from build123d import *

# Parameters (mm, degrees)
F0_R      = 11.5
F1_DEPTH  = 2
F3_DEPTH  = 5
F5_DEPTH  = 10.5
F6_W      = 0.8
F6_H      = 5
F7_DEPTH  = 5
F8_R      = 8.8
F9_DEPTH  = 6
F11_R     = 2
F12_SIZE  = 0.75
F13_R     = 0.9
F14_DEPTH = 21.9495823706


# Not quite as in the source:
# - a fillet or chamfer that OpenCascade refuses, or shapes differently, is made with other operations: its cross-section is extruded or revolved along the edge and cut away or added


with BuildPart() as f1:
    # F0 (on Top) → F1 (new body)
    with BuildSketch(Plane.XY):
        Circle(F0_R)
    extrude(amount=F1_DEPTH)

    # F2 (on face) → F3 (join)
    with BuildSketch(Plane(origin=(0, 0, 0), x_dir=(1, 0, 0), z_dir=(0, 0, -1))):
        with BuildLine():
            Line((-9.05, -2), (-9.05, -3.6276714294))
            ThreePointArc((-9.05, -3.6276714294), (0, -9.75), (9.05, -3.6276714294))
            Line((9.05, -3.6276714294), (9.05, -2))
            Line((9.05, -2), (9.05, 2))
            Line((9.05, 2), (9.05, 3.6276714294))
            ThreePointArc((9.05, 3.6276714294), (5.8706571109, 7.7844643416), (1, 9.6985823706))
            Line((1, 9.6985823706), (1, 10.4485823706))
            Line((1, 10.4485823706), (-1, 10.4485823706))
            Line((-1, 10.4485823706), (-1, 9.6985823706))
            ThreePointArc((-1, 9.6985823706), (-5.8706571109, 7.7844643416), (-9.05, 3.6276714294))
            Line((-9.05, 3.6276714294), (-9.05, 2))
            Line((-9.05, 2), (-9.05, -2))
        make_face()
        with BuildLine():
            Line((-9.542667342, -2), (-9.05, -2))
            Line((-9.05, -2), (-9.05, 2))
            Line((-9.05, 2), (-9.542667342, 2))
            ThreePointArc((-9.542667342, 2), (-9.75, 0), (-9.542667342, -2))
        make_face()
        with BuildLine():
            Line((9.05, 2), (9.05, -2))
            Line((9.05, -2), (9.542667342, -2))
            ThreePointArc((9.542667342, -2), (9.75, 0), (9.542667342, 2))
            Line((9.542667342, 2), (9.05, 2))
        make_face()
    extrude(amount=F3_DEPTH)

    # F4 (on face) → F5 (join)
    with BuildSketch(Plane(origin=(0, 0, -5), x_dir=(1, 0, 0), z_dir=(0, 0, -1))):
        with BuildLine():
            Line((6.5, 5.35), (-6.5, 5.35))
            ThreePointArc((-6.5, 5.35), (-7.9142135624, 4.7642135624), (-8.5, 3.35))
            Line((-8.5, 3.35), (-8.5, -3.35))
            ThreePointArc((-8.5, -3.35), (-7.9142135624, -4.7642135624), (-6.5, -5.35))
            Line((-6.5, -5.35), (6.5, -5.35))
            ThreePointArc((6.5, -5.35), (7.9142135624, -4.7642135624), (8.5, -3.35))
            Line((8.5, -3.35), (8.5, 3.35))
            ThreePointArc((8.5, 3.35), (7.9142135624, 4.7642135624), (6.5, 5.35))
        make_face()
    extrude(amount=F5_DEPTH)

    # F6 (on face) → F7 (cut)
    with BuildSketch(Plane(origin=(0, 0, -15.5), x_dir=(1, 0, 0), z_dir=(0, 0, -1))):
        Rectangle(F6_W, F6_H)
        with Locations((-7.1, 0)):
            Rectangle(F6_W, F6_H)
        with Locations((7.1, 0)):
            Rectangle(F6_W, F6_H)
    extrude(amount=-F7_DEPTH, mode=Mode.SUBTRACT)

    # F8 (on face) → F9 (cut)
    with BuildSketch(Plane.XY.offset(2)):
        Circle(F8_R)
    extrude(amount=-F9_DEPTH, mode=Mode.SUBTRACT)

    # F10: chamfer of 2.8 x 1 on 1 edges, made by hand

    # F10_s1 → F10_t2 (revolve, cut)
    with BuildSketch(Plane.XZ):
        Polygon((11.5, 1), (8.7, 2), (11.5, 2), align=None)
    revolve(axis=Axis((0, 0, 2), (0, 0, 1)), mode=Mode.SUBTRACT)

    # F11
    f11_edges = [f1.edges().sort_by_distance(p)[0] for p in [
        (-9.05, 3.627671, -2.5),
        (-9.05, -3.627671, -2.5),
        (9.05, -3.627671, -2.5),
        (9.05, 3.627671, -2.5),
    ]]
    fillet(f11_edges, radius=F11_R)

    # F12
    f12_edges = [f1.edges().sort_by_distance(p)[0] for p in [
        (0, -10.448582, -5),
    ]]
    chamfer(f12_edges, length=F12_SIZE)

    # F13 (on face) → F14 (cut, through all)
    with BuildSketch(Plane.XZ.offset(10.4485823706)):
        with Locations((0, -1.4)):
            Circle(F13_R)
    extrude(amount=-F14_DEPTH, mode=Mode.SUBTRACT)


solid = f1.part
The listing builds one solid part. Answer for the finished solid, in the listing's coordinates (mm). A direction names the side the tool comes from. Coordinates: 2 decimals unless noted, no trailing zeros. Loops run counter-clockwise (first coordinate to the right, second up) from the corner with the lowest first, then second, coordinate; pieces in that order, holes last. Notation, with made-up numbers: (-39, 82.25) -> (6, 82.25) arc R19 cw to (6, 91.25) -> close; hole circle Ø11 at (29.25, -29.5). An arc over 180 degrees is marked (long way). Write item = value, one per line. Start each with the question number.
1) A cutting plane is placed at B-B (z = -1.4). Give the vertices of the cut face in (x, y), then the cut area to 3 significant figures.
2) A cutting plane is placed at A-A (x = 0). Count the separate pieces of the cut face and the enclosed holes in it, then the cut area to 3 significant figures.
3) The mould has two halves that part along X. Classify faces 1 (the face through (-0.16, 9.75, -2.46)), 2 (the face through (9.003, -3.65, -2.535)), 3 (the face through (0, 5.35, -10)), 4 (the face through (-6.7, 0, -13)): released by +X, released by -X, zero draft, split by the parting line, or undercut.
4) Straight lines are drawn through the part: line 1 (Z direction, x = 5, y = -3); line 2 (X direction, y = -0.5, z = -6.5); line 3 (Y direction, x = 2.5, z = -13). For each, find the intervals that lie inside material, in ascending order. Write a range as from..to.
5) Given pin 1 Ø0.9 at (x, z) = (-7.5, -13.5) entering from +Y; pin 2 Ø5 at (y, z) = (-5.5, -6.5) entering from -X; pin 3 Ø1.5 at (y, z) = (-0.5, -11.5) entering from +X, each flat-ended and moving along its own axis, determine where each tip first touches the part or whether it passes through.
6) A tool of negligible diameter and unlimited length cuts with its end or side. For faces 5 (the face through (5.74, -7.88, -2.46)), 6 (the face through (-1.146, 8.725, -0.976)), 7 (the face through (7, 2.5, -13)), from which of +Z, -Z, +X, -X, +Y, -Y can it reach the whole face along a straight path? Write none if from no direction.
7) A cutting plane is placed at C-C (y = 0). Give the vertices of the cut face in (x, z).
Responses:
q1.outline = (-9.54, -2) -> (-9.05, -2) -> (-9.05, -3.22) arc R2 ccw to (-8.87, -4.05) arc R9.75 ccw to (-1, -9.7) -> (-1, -10.45) -> (-0.9, -10.45) -> (-0.9, -8.75) arc R8.8 cw to (-0.9, 8.75) -> (-0.9, 9.71) arc R9.75 ccw to (-8.87, 4.05) arc R2 ccw to (-9.05, 3.22) -> (-9.05, 2) -> (-9.54, 2) arc R9.75 ccw to start; (0.9, -10.45) -> (1, -10.45) -> (1, -9.7) arc R9.75 ccw to (8.87, -4.05) arc R2 ccw to (9.05, -3.22) -> (9.05, -2) -> (9.54, -2) arc R9.75 ccw to (9.54, 2) -> (9.05, 2) -> (9.05, 3.22) arc R2 ccw to (8.87, 4.05) arc R9.75 ccw to (0.9, 9.71) -> (0.9, 8.75) arc R8.8 cw to (0.9, -8.75) -> close
q1.area = 50.3 mm²
q2.separate_pieces = 3
q2.enclosed_holes = 0
q2.area = 121 mm²
q3.face_1 = split by the parting line
q3.face_2 = released by +X
q3.face_3 = zero draft
q3.face_4 = undercut
q4.line_1 = -15.5..-4
q4.line_2 = -8.5..8.5
q4.line_3 = -5.35..5.35
q5.pin_1 = 5.27
q5.pin_2 = -9.03
q5.pin_3 = 8.5
q6.face_5 = -Z, +X, -Y
q6.face_6 = +Z
q6.face_7 = -Z
q7.outline = (-11.5, 0) -> (-9.75, 0) -> (-9.75, -5) -> (-8.5, -5) -> (-8.5, -15.5) -> (-7.5, -15.5) -> (-7.5, -10.5) -> (-6.7, -10.5) -> (-6.7, -15.5) -> (-0.4, -15.5) -> (-0.4, -10.5) -> (0.4, -10.5) -> (0.4, -15.5) -> (6.7, -15.5) -> (6.7, -10.5) -> (7.5, -10.5) -> (7.5, -15.5) -> (8.5, -15.5) -> (8.5, -5) -> (9.75, -5) -> (9.75, 0) -> (11.5, 0) -> (11.5, 1) -> (8.8, 1.96) -> (8.8, -4) -> (-8.8, -4) -> (-8.8, 1.96) -> (-11.5, 1) -> close
